Design review of the part shown in the three views and the two pictorial views. Dimensions are in mm from the part's minimum x, y and z. A direction names the side the tool comes from. Round coordinates to 2 decimals unless told otherwise and drop trailing zeros. Write each loop counter-clockwise with the first axis right and the second up, starting at its lowest first coordinate (ties: lowest second). Pieces come first, ordered by that corner, then holes. Notation, with made-up numbers: (28, 87) - (75, 87) arc R19 cw to (75, 107) - close; hole circle Ø4 at (62.5, -0.75). An arc over 180 degrees is marked (long way). Use one line per item in the form item = value.
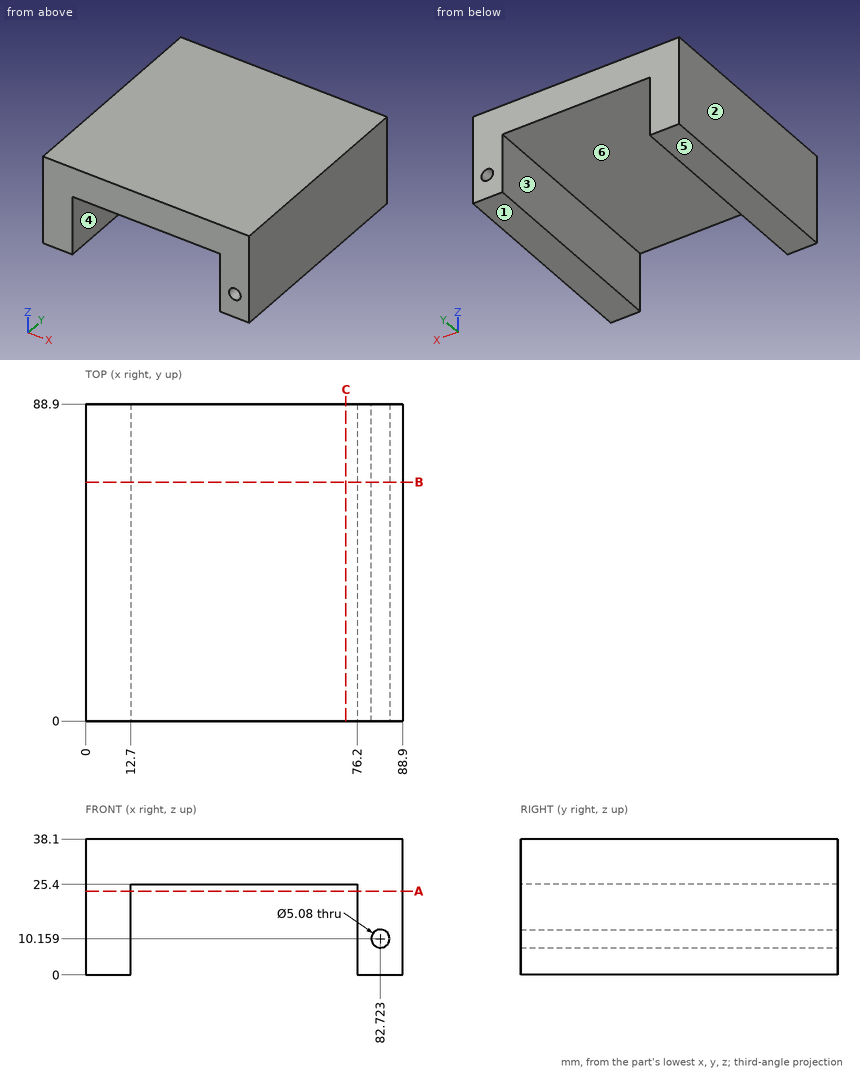
(1) Machinability: for the marked faces 5 and 6, which of the approach directions +Z, -Z, +X, -X, +Y, -Y give a long, thin tool a straight path to every point of the face, cutting with its end or side? Answer none if there is none.
Geometry results:
face_5 = -Z, +X, -X, +Y, -Y
face_6 = -Z, +Y, -Y
(2) Add section C-C on x = 73. Write out the cut boundary in (y, z).
Geometry results:
outline = (0, 25.4) - (88.9, 25.4) - (88.9, 38.1) - (0, 38.1) - close
(3) To check wall thickness, follow L1, parallel to X at y = 71, z = 19; L2, parallel to X at y = 20, z = 9 (1 decimal); L3, parallel to X at y = 18, z = 11.5 (1 decimal). State the ranges of each line that lie inside material, in increasing order.
Geometry results:
L1 = 0 to 12.7, 76.2 to 88.9
L2 = 0 to 12.7, 76.2 to 80.5, 85 to 88.9
L3 = 0 to 12.7, 76.2 to 80.6, 84.9 to 88.9
(4) The part is to be moulded in two halves that separate along X. For the marked faces 1, 2, 3 and 4, say which applies: +X half, -X half, draft (parallel to the pull), parting line (faces both ways), or undercut.
Geometry results:
face_1 = draft
face_2 = -X half
face_3 = undercut
face_4 = undercut
(5) Add section A-A on z = 23.5. Write out the cut boundary in (x, y).
Geometry results:
outline = (0, 0) - (12.7, 0) - (12.7, 88.9) - (0, 88.9) - close; (76.2, 0) - (88.9, 0) - (88.9, 88.9) - (76.2, 88.9) - close
(6) Add section B-B on y = 67. Write out the cut boundary in (x, z).
Geometry results:
outline = (0, 0) - (12.7, 0) - (12.7, 25.4) - (76.2, 25.4) - (76.2, 0) - (88.9, 0) - (88.9, 38.1) - (0, 38.1) - close; hole circle Ø5.08 at (82.72, 10.16)
(7) Insertion check: P1, Ø20.5, axis at y = 55, z = 14, coming from the -X side; P2, Ø10, axis at x = 42, z = 20, coming from the -Y side. Each pin has a flat end and moves straight along its axis. Give the tip position at first contact, or say it passes through.
Geometry results:
P1 = 0
P2 = through
